Autodesk Inventor part; units mm, degrees
ref_plane "YZ Plane" through (0, 0, 0) normal (1, 0, 0) x (0, 1, 0)
ref_plane "XZ Plane" through (0, 0, 0) normal (0, 1, 0) x (-1, 0, 0)
ref_plane "XY Plane" through (0, 0, 0) normal (0, 0, 1) x (1, 0, 0)
sketch "Sketch1" plane through (0, 0, 0) normal (0, 0, 1) x (1, 0, 0)
  line L0 (0, 0) -> (63.5, 0)
  line L1 (63.5, 0) -> (63.5, -12.7)
  line L2 (63.5, -12.7) -> (12.7, -12.7)
  line L3 (12.7, -12.7) -> (12.7, -33.02)
  line L4 (12.7, -33.02) -> (-43.18, -33.02)
  line L5 (-43.18, -33.02) -> (-43.18, -20.32)
  line L6 (-43.18, -20.32) -> (0, -20.32)
  line L7 (0, -20.32) -> (0, 0)
  dimension "d0" = 12.7
  dimension "d2" = 12.7
  dimension "d3" = 12.7
  dimension "d4" = 43.18
  dimension "d5" = 20.32
  dimension "d22" = 50.8
extrude "Extrusion1" add sketch "Sketch1" along normal blind 17.78
sketch "Sketch2" plane through (0, 0, 0) normal (0, 1, 0) x (1, 0, 0)
  line L0 (63.5, 0) -> (63.5, -17.78)
  line L1 (0, 0) -> (0, -17.78)
  line L2 (0, -8.89) -> (63.5, -8.89) construction
  point P0 (50.8, -8.89)
  point P1 (25.4, -8.89)
  dimension "d8" = 12.7
  dimension "d9" = 25.4
hole "Hole1" at (50.8, 0, 8.89) at (25.4, 0, 8.89) direction (0, -1, 0) diameter 4.4958 end through all
sketch "Sketch3" plane through (-43.18, -33.02, 0) normal (0, -1, 0) x (1, 0, 0)
  line L0 (0, 0) -> (0, 17.78)
  line L1 (55.88, 0) -> (55.88, 17.78)
  line L2 (0, 8.89) -> (55.88, 8.89) construction
  arc A0 (11.5583, 7.62) -> (11.5583, 10.16) centre (17.78, 8.89) ccw
  line L3 (11.5583, 10.16) -> (0, 10.16)
  line L4 (0, 7.62) -> (11.5583, 7.62)
  line L5 (0, 10.16) -> (0, 7.62)
  point P0 (43.18, 0)
  dimension "d17" = 12.7
  dimension "d18" = 17.78
  dimension "d19" = 2.54
extrude "Extrusion2" cut sketch "Sketch3" against normal up to next
sketch "Sketch4" plane through (0, 0, 17.78) normal (0, 0, 1) x (1, 0, 0)
  line L0 (-43.18, -33.02) -> (-43.18, -20.32)
  line L1 (12.7, -12.7) -> (12.7, -33.02)
  line L2 (-43.18, -26.67) -> (12.7, -26.67) construction
  point P0 (-36.83, -26.67)
  dimension "d23" = 6.35
hole "Hole3" at (-36.83, -26.67, 17.78) direction (0, 0, -1) diameter 3.81 end up to surface
hole "Hole4" at (-36.83, -26.67, 17.78) direction (0, 0, -1) diameter 2.6416 end through all
sketch "Sketch6" plane through (-43.18, -33.02, 0) normal (0, -1, 0) x (1, 0, 0)
  line L0 (0, 10.16) -> (11.5583, 10.16)
  arc A0 (11.5583, 7.62) -> (11.5583, 10.16) centre (17.78, 8.89) ccw
  line L1 (11.5583, 7.62) -> (0, 7.62)
  line L2 (0, 0) -> (0, 7.62)
  line L3 (55.88, 0) -> (0, 0)
  line L4 (55.88, 0) -> (55.88, 17.78)
  line L5 (55.88, 17.78) -> (0, 17.78)
  line L6 (0, 10.16) -> (0, 17.78)
  line L7 (55.88, 17.78) -> (30.48, 17.78)
  line L8 (30.48, 17.78) -> (30.48, 12.7)
  line L9 (30.48, 12.7) -> (55.88, 12.7)
  line L10 (55.88, 12.7) -> (55.88, 17.78)
  line L11 (55.88, 0) -> (30.48, 0)
  line L12 (30.48, 0) -> (30.48, 5.08)
  line L13 (30.48, 5.08) -> (55.88, 5.08)
  line L14 (55.88, 5.08) -> (55.88, 0)
  point P0 (43.18, 0)
  dimension "d56" = 5.08
  dimension "d57" = 25.4
  dimension "d58" = 5.08
  dimension "d59" = 25.4
extrude "Extrusion3" add sketch "Sketch6" along normal blind 19.05 contours L5 L4 L9 L8 | L12 L13 L4 L3
sketch "Sketch8" plane through (0, 0, 17.78) normal (0, 0, 1) x (1, 0, 0)
  line L0 (-12.7, -33.02) -> (-43.18, -33.02)
  line L1 (12.7, -12.7) -> (12.7, -52.07)
  point P0 (0, 0)
  point P1 (7.112, -45.72)
  point P2 (-2.286, -45.72)
  dimension "d66" = 12.7
  dimension "d67" = 12.7
  dimension "d68" = 14.986
  dimension "d69" = 9.398
hole "Hole6" at (7.112, -45.72, 17.78) at (-2.286, -45.72, 17.78) direction (0, 0, -1) diameter 5.08 end up to surface
hole "Hole7" at (-2.286, -45.72, 17.78) direction (0, 0, -1) diameter 1.7018 end through all
hole "Hole8" at (7.112, -45.72, 17.78) direction (0, 0, -1) diameter 1.7018 end through all
sketch "Sketch9" plane through (-43.18, -20.32, 0) normal (0, 1, 0) x (1, 0, 0)
  line L0 (11.5583, -10.16) -> (0, -10.16)
  line L1 (0, -10.16) -> (0, -17.78)
  line L2 (0, -17.78) -> (43.18, -17.78)
  line L3 (43.18, 0) -> (43.18, -17.78)
  line L4 (0, 0) -> (43.18, 0)
  line L5 (0, 0) -> (0, -7.62)
  line L6 (0, -7.62) -> (11.5583, -7.62)
  arc A0 (11.5583, -10.16) -> (11.5583, -7.62) centre (17.78, -8.89) ccw
  point P0 (36.195, -8.89)
  dimension "d95" = 18.415
hole "Hole9" at (-6.985, -20.32, 8.89) direction (0, -1, 0) diameter 5.08 end through all
properties part number "J001396" material "ALUMINUM, 6061-T651"
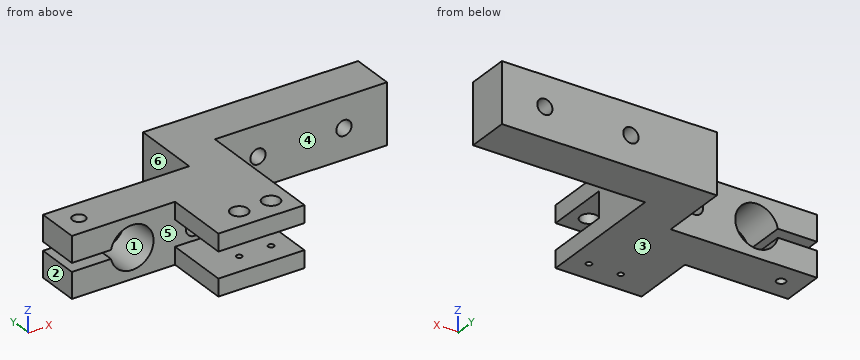
CAD build for the part. Positions are in the model's coordinates, mm. Face numbers are marked on the shaded views. A direction names the side the tool comes from. Round coordinates to 2 decimals unless told otherwise and drop trailing zeros. Loops run counter-clockwise (first coordinate to the right, second up) from the corner with the lowest first, then second, coordinate; pieces in that order, holes last. Notation, with made-up numbers: (63, 0.5) - (85, 0.5) arc R12 ccw to (85, 17.5) - close; hole circle Ø11 at (-12, 22.25). An arc over 180 degrees is marked (long way). Put each result on its own line as item: value.
1. Pin check, flat tips, straight feed: P1, Ø9, axis at y = -24, z = 6, coming from the +X side; P2, Ø2, axis at x = 7.112, y = -45.72, coming from the +Z side; P3, Ø6, axis at y = -16, z = 2, coming from the -X side. Stop position of each tip, or through.
Geometry check:
P1: x = 12.7
P2: z = 5.08
P3: x = 0
2. 3-axis set-ups, long thin cutter, end or side, ignore diameter. For the marked faces 4, 5 and 6: which of +Z, -Z, +X, -X, +Y, -Y reach the whole face in a straight line?
Geometry check:
face 4: +Z, -Z, +X, -Y
face 5: -X, -Y
face 6: +Z, -Z, -X, +Y
3. Slice it at C-C on z = 14. List the corners of the cut face in (x, y) (3 decimals).
Geometry check:
outline: (-43.18, -33.02) - (-29.17, -33.02) - (-29.17, -20.32) - (-43.18, -20.32) - close; (-21.63, -33.02) - (-12.7, -33.02) - (-12.7, -52.07) - (12.7, -52.07) - (12.7, -12.7) - (63.5, -12.7) - (63.5, 0) - (0, 0) - (0, -20.32) - (-21.63, -20.32) - close; hole circle Ø3.81 at (-36.83, -26.67); hole circle Ø5.08 at (-2.286, -45.72); hole circle Ø5.08 at (7.112, -45.72)
4. Slice it at B-B on y = -34.5. List the corners of the cut face in (x, z), and give its area (3 significant figures).
Geometry check:
outline: (-12.7, 0) - (12.7, 0) - (12.7, 5.08) - (-12.7, 5.08) - close; (-12.7, 12.7) - (12.7, 12.7) - (12.7, 17.78) - (-12.7, 17.78) - close
area: 258 mm²
5. Two-plate mould, pull along Z, no slides. Class the marked faces 1, 2 and 3: released by +Z, released by -Z, zero draft, split by the parting line, or undercut.
Geometry check:
face 1: undercut
face 2: zero draft
face 3: released by -Z
6. Wall check: line 1 (X direction, y = -3, z = 8.89); line 2 (X direction, y = -45.72, z = 15.7); line 3 (Y direction, x = -36.83, z = 5.25). Give the ranges that are in metal, low to high.
Geometry check:
line 1: 0 to 23.15, 27.65 to 48.55, 53.05 to 63.5
line 2: -12.7 to -4.83, 0.25 to 4.57, 9.65 to 12.7
line 3: -33.02 to -27.99, -25.35 to -20.32
7. Slice it at D-D on z = 8.89. List the corners of the cut face in (x, y) (3 decimals), and give its area (3 significant figures).
Geometry check:
outline: (-19.05, -33.02) - (-9.525, -33.02) - (-9.525, -20.32) - (-19.05, -20.32) - close; (-4.445, -33.02) - (12.7, -33.02) - (12.7, -12.7) - (23.152, -12.7) - (23.152, 0) - (0, 0) - (0, -20.32) - (-4.445, -20.32) - close; (27.648, -12.7) - (48.552, -12.7) - (48.552, 0) - (27.648, 0) - close; (53.048, -12.7) - (63.5, -12.7) - (63.5, 0) - (53.048, 0) - close
area: 1,130 mm²
8. Slice it at A-A on x = -25.4. List the corners of the cut face in (y, z), and give its area (3 significant figures).
Geometry check:
outline: (-33.02, 0) - (-20.32, 0) - (-20.32, 2.54) - (-33.02, 2.54) - close; (-33.02, 15.24) - (-20.32, 15.24) - (-20.32, 17.78) - (-33.02, 17.78) - close
area: 64.5 mm²
